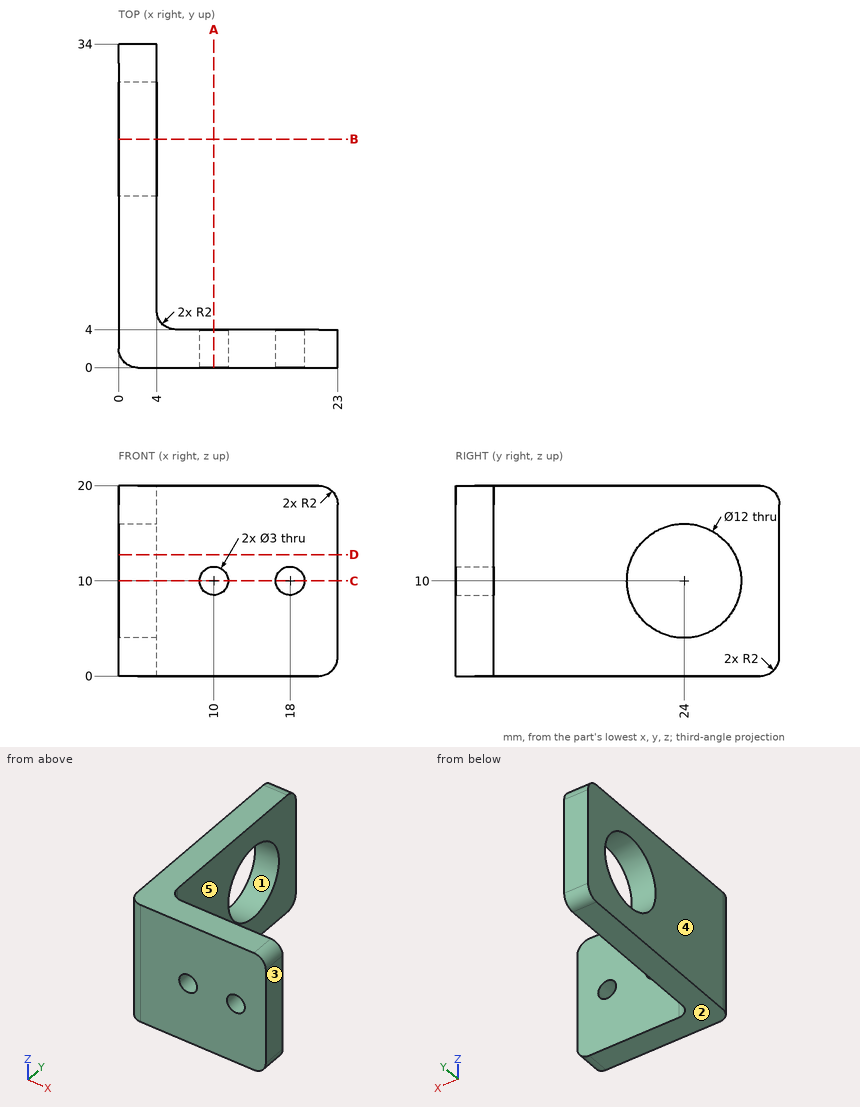
Could you check a few things on this drawing? It's one solid part, dimensions in mm from its lowest x, y, z. A direction names the side the tool comes from. Round coordinates to 2 decimals unless told otherwise and drop trailing zeros. Order: outer loops, then holes, each group sorted by start corner. A loop starts at its lowest first (then second) coordinate and runs counter-clockwise, first axis right, second up. Notation, with made-up numbers: M -24.5,-7.5 L -9.5,-7.5 A33 cw -9.5,31.5 Z; hole C 58,-19.5 d2. An arc over 180 degrees is marked long. Use a Markdown table: item, result.
1) Imagine slicing it at D-D (z = 12.75). List the corners of the cut face in (x, y) for me.
Geometry says:
| item | result |
|---|---|
| outline | M 0,2 A2 ccw 2,0 L 23,0 L 23,4 L 6,4 A2 cw 4,6 L 4,18.67 L 0,18.67 Z; M 0,29.33 L 4,29.33 L 4,34 L 0,34 Z |
2) Imagine slicing it at A-A (x = 10). List the corners of the cut face in (y, z) for me, then the cut area to 3 significant figures.
Geometry says:
| item | result |
|---|---|
| outline | M 0,0 L 4,0 L 4,8.5 L 0,8.5 Z; M 0,11.5 L 4,11.5 L 4,20 L 0,20 Z |
| area | 68.0 mm² |
3) On a 3-axis mill with a long thin cutter (end or side, diameter ignored), from which of +Z, -Z, +X, -X, +Y, -Y can I reach the whole of each face in a straight line? I mean the marked faces 4 and 5. Say none if no direction works.
Geometry says:
| item | result |
|---|---|
| face 4 | +Z, -Z, -X, +Y, -Y |
| face 5 | +Z, -Z, +X, +Y |
4) Imagine slicing it at C-C (z = 10). List the corners of the cut face in (x, y) for me, then the cut area to 3 significant figures.
Geometry says:
| item | result |
|---|---|
| outline | M 0,2 A2 ccw 2,0 L 8.5,0 L 8.5,4 L 6,4 A2 cw 4,6 L 4,18 L 0,18 Z; M 0,30 L 4,30 L 4,34 L 0,34 Z; M 11.5,0 L 16.5,0 L 16.5,4 L 11.5,4 Z; M 19.5,0 L 23,0 L 23,4 L 19.5,4 Z |
| area | 140 mm² |
5) I'm going to push flat-ended pins straight in: P1, Ø8, axis at x = 18, z = 11.5, coming from the +Y side; P2, Ø2, axis at y = 13.5, z = 4, coming from the +X side. Where does each tip first touch, or does it pass through?
Geometry says:
| item | result |
|---|---|
| P1 | stops at y = 4 |
| P2 | stops at x = 4 |
6) If we mould it in two halves opening along Z, with no side actions, what happens to the marked faces 1, 2 and 3? For each: +Z half, -Z half, draft (parallel to the pull), parting line (faces both ways), or undercut.
Geometry says:
| item | result |
|---|---|
| face 1 | undercut |
| face 2 | -Z half |
| face 3 | draft |
7) Imagine slicing it at B-B (y = 24). List the corners of the cut face in (x, z) for me.
Geometry says:
| item | result |
|---|---|
| outline | M 0,0 L 4,0 L 4,4 L 0,4 Z; M 0,16 L 4,16 L 4,20 L 0,20 Z |
8) If I drill on line 1 along X through (y, z) = (32.5, 11); line 2 along Z through (x, y) = (18, 2.8), over which ranges is the centre line in solid material (lowest first)?
Geometry says:
| item | result |
|---|---|
| line 1 | x = 0 to 4 |
| line 2 | z = 0 to 8.5, 11.5 to 20 |
